```python
from build123d import *

# Parameters (mm, degrees)
BOSS_EXTRUDE1_DEPTH = 5
BOSS_EXTRUDE3_DEPTH = 1
SKETCH4_R           = 3.555
BOSS_EXTRUDE4_DEPTH = 2.5
SKETCH5_R           = 1
CUT_EXTRUDE3_DEPTH  = 0.15
SKETCH3_R           = 2.5
CUT_EXTRUDE5_DEPTH  = 9.5


with BuildPart() as part:
    # Sketch2 → Boss-Extrude1 (new body)
    with BuildSketch(Plane(origin=(0, 0, 0), x_dir=(0, 0, -1), z_dir=(1, 0, 0))):
        Polygon((3.919437566, -2.29861752), (3.950379949, 2.245023741), (0.030942383, 4.54364126), (-3.919437566, 2.29861752), (-3.950379949, -2.245023741), (-0.030942383, -4.54364126), align=None)
    extrude(amount=BOSS_EXTRUDE1_DEPTH)

    # Sketch6 → Boss-Extrude3 (add)
    with BuildSketch(Plane.ZY):
        with BuildLine():
            Line((4.699218, 1.737080939), (4.71082912, 0.032080939))
            Line((4.71082912, 0.032080939), (4.722440239, -1.672919061))
            ThreePointArc((4.722440239, -1.672919061), (-5.009883831, -0.034117514), (4.699218, 1.737080939))
        make_face()
    extrude(amount=BOSS_EXTRUDE3_DEPTH)

    # Sketch4 → Boss-Extrude4 (add)
    with BuildSketch(Plane.ZY.offset(1)):
        Circle(SKETCH4_R)
    extrude(amount=BOSS_EXTRUDE4_DEPTH)

    # Sketch5 → Cut-Extrude3 (cut)
    with BuildSketch(Plane(origin=(0, 0.02679689, 3.934908757), x_dir=(1, 0, 0), z_dir=(0, -0.006809883, -0.999976812))):
        with Locations((2.5, 0)):
            Circle(SKETCH5_R)
    extrude(amount=CUT_EXTRUDE3_DEPTH, mode=Mode.SUBTRACT)

    # Sketch3 → Cut-Extrude5 (cut, through all)
    with BuildSketch(Plane.ZY.offset(3.5)):
        with Locations((0.79, 0)):
            Circle(SKETCH3_R)
    extrude(amount=-CUT_EXTRUDE5_DEPTH, mode=Mode.SUBTRACT)

    # Sketch7 → Cut-Revolve1 (revolve, cut)
    with BuildSketch(Plane.XY):
        Polygon((4.422649731, 4.54364126), (5, 3.54364126), (9.422649731, 3.54364126), (9.422649731, 8.54364126), (4.422649731, 8.54364126), align=None)
    revolve(axis=Axis((0, 0, 0), (1, 0, 0)), mode=Mode.SUBTRACT)


solid = part.part
```
Check sheet for the modelled part. Datum: model origin and axes. Units: mm. A direction names the side the tool comes from. Coordinates: 2 decimals unless noted, no trailing zeros. Order: outer loops, then holes, each group sorted by start corner. A loop starts at its lowest first (then second) coordinate and runs counter-clockwise, first axis right, second up. Notation, with made-up numbers: M 49,-19.5 L 79,-19.5 A26 cw 79,16.5 Z; hole C 8,-10 d1. An arc over 180 degrees is marked long. Write each question's results on one line, items separated by ' | '. Start each with the question number.
1. Material ranges on probe 1 along Y at (x, z) = (2.5, 0.79); probe 2 along Z at (x, y) = (3, 0.5); probe 3 along Z at (x, y) = (1, 0.25), recorded low to high.
2. Cross-section at B-B on x = 2.75. Record the cut outline in (y, z), and give its area (3 significant figures).
3. Mould release check, pull along Y, two halves, no side actions. Record for faces 4 (the face through (5, 0, -2)), 5 (the face through (-2.23, 1.07, 3.39)), 6 (the face through (0.69, -2.44, 0.25)): +Y half, -Y half, draft (parallel to the pull), parting line (faces both ways), or undercut.
4. Cross-section at A-A on x = 1. Record the cut outline in (y, z).
5. Go/stop test with flat-tipped pins: P1, Ø1, axis at x = -0.5, z = 2.5, coming from the +Y side; P2, Ø4, axis at x = 2.5, y = -2, coming from the +Z side; P3, Ø1, axis at x = -2.5, y = 3.5, coming from the +Z side. Record where each tip stops, or that it passes through.
6. Access from +Z, -Z, +X, -X, +Y, -Y to the whole of each face (thin tool, end or side, straight path). Record for faces 1 (the face through (-1, 2.3, 3.2)), 2 (the face through (2.354, 3.378, -2.018)), 3 (the face through (2.354, 3.437, 1.917)).
Checks:
1) probe 1: y = -4.1 to -2.5, 2.5 to 4.08 | probe 2: z = -3.94 to -1.66, 3.24 to 3.78 | probe 3: z = -3.94 to -1.7, 3.28 to 3.93
2) outline: M -4.54,0.03 L -2.3,-3.92 L 2.25,-3.95 L 4.54,-0.03 L 2.3,3.92 L 1,3.93 L 0.99,3.78 L -0.94,3.79 L -0.94,3.94 L -2.25,3.95 Z; hole C 0,0.79 d5 | area: 33.7 mm²
3) face 4: draft | face 5: parting line | face 6: undercut
4) outline: M -4.54,0.03 L -2.3,-3.92 L 2.25,-3.95 L 4.54,-0.03 L 2.3,3.92 L -2.25,3.95 Z; hole C 0,0.79 d5
5) P1: stops at y = 4.59 | P2: stops at z = 3.95 | P3: stops at z = 1.91
6) face 1: -X | face 2: -Z, +X, +Y | face 3: +Z, +X, +Y
